Read the model definition and answer for the solid it produces. Units are mm, in the model's axes. A direction names the side the tool comes from. Coordinates: 2 decimals unless noted, no trailing zeros. Loops run counter-clockwise (first coordinate to the right, second up) from the corner with the lowest first, then second, coordinate; pieces in that order, holes last. Notation, with made-up numbers: M 30.5,-38 L 36.5,-38 A27 ccw 36.5,-12 Z; hole C 19,-3 d8. An arc over 180 degrees is marked long. One line per item, written item: value. Start each with the question number.
1. Consider probe 1 along Y at (x, z) = (-64.5, 0.15); probe 2 along Z at (x, y) = (-74, -3.75); probe 3 along Y at (x, z) = (-100, 0.3). Determine where each line is inside the solid, lowest interval first.
2. For faces 1 (the face through (-93.713, -3.228, -0.032)), 2 (the face through (-45.7, 3.5, 0.1)), 3 (the face through (-46, 0, 0)), determine the directions among +Z, -Z, +X, -X, +Y, -Y from which every point of the face is accessible in a straight line to the end or side of a thin tool.
3. Determine the mould class of faces 4 (the face through (-44.453, -6.078, 0.069)), 5 (the face through (0, 1, 0)), 6 (the face through (-93.57, 0.63, -0.03)) for opening direction X: +X half, -X half, draft (parallel to the pull), parting line (faces both ways), or undercut.
4. Flat-ended cylindrical pins translate along their axes: pin 1 (1.4 mm diameter, centred on x = -55, z = 0, fed in from -Y); pin 2 (1.4 mm diameter, centred on x = -34, z = 0.5, fed in from +Y); pin 3 (1 mm diameter, centred on y = -1, z = 1, fed in from +X). Find the tip coordinate at first contact, or state that the pin passes through.
5. The part is cut by section A-A (x = -49). Write down the section's boundary in (y, z), then the cut area to 3 significant figures.
6. The part is cut by section B-B (z = 0.1). Write down the section's boundary in (x, y).
```python
from build123d import *


with BuildPart() as part:
    # Sweep1: sweep along a path in Sketch1
    with BuildLine(Plane.XY) as sweep1_path:
        Line((0, 0), (-90.078432584, 0))
        ThreePointArc((-90.078432584, 0), (-93.613966489, 0.645856533), (-96.692810861, 2.5))
        ThreePointArc((-96.692810861, 2.5), (-104.999960358, -1.230089771), (-96.72278085, -5.026219624))
        ThreePointArc((-96.72278085, -5.026219624), (-93.666599798, -3.210510909), (-90.168342551, -2.578658871))
        Line((-90.168342551, -2.578658871), (0, -2.578658871))
    # Sketch2 → Sweep1 (sweep)
    with BuildSketch(Plane(origin=(0, 0, 0), x_dir=(0, 0, -1), z_dir=(1, 0, 0))):
        with BuildLine():
            Line((2.291287847, 0), (-2.291287847, 0))
            ThreePointArc((-2.291287847, 0), (0, 3.5), (2.291287847, 0))
        make_face()
    sweep(path=sweep1_path.line)


solid = part.part
```
Answer block:
1. probe 1: y = -6.07 to -2.58, 0 to 3.5
1. probe 2: z = -2.49 to 2.49
1. probe 3: y = -9.73 to -6.25, 3.75 to 7.23
2. face 1: +Z, -Z
2. face 2: +X
2. face 3: +Z, -Z, +X
3. face 4: draft
3. face 5: +X half
3. face 6: undercut
4. pin 1: stops at y = -6.08
4. pin 2: stops at y = 3.5
4. pin 3: stops at x = -104.94
5. outline: M -2.58,-2.29 L -2.58,2.29 A2.5 ccw long Z; M 0,-2.29 A2.5 ccw long 0,2.29 Z
5. area: 29.4 mm2
6. outline: M -96.72,-5.03 A5 cw long -96.69,2.5 A10 ccw -90.08,0 L 0,0 L 0,3.5 L -90.08,3.5 A6.5 cw -94.38,5.12 A8.5 ccw long -94.43,-7.67 A6.5 cw -90.17,-6.08 L 0,-6.08 L 0,-2.58 L -90.17,-2.58 A10 ccw Z
